from build123d import *

# Parameters (mm, degrees)
SKETCH1_W           = 422.275
SKETCH1_H           = 241.3
BOSS_EXTRUDE1_DEPTH = 19.05
CUT_EXTRUDE1_REACH  = 245.923
SKETCH2_W           = 231.775
SKETCH2_H           = 65.151
CUT_EXTRUDE2_REACH  = 323.197
SKETCH3_W           = 14.2875
SKETCH3_H           = 3.175
CUT_EXTRUDE3_REACH  = 323.197
SKETCH4_W           = 13.49375
SKETCH4_H           = 3.175
FILLET1_R           = 63.5
CUT_EXTRUDE4_REACH  = 323.197
SKETCH5_W           = 13.49375
SKETCH5_H           = 9.525
CHAMFER1_SIZE       = 3.175
CHAMFER1_SIZE2      = 11.849261314


with BuildPart() as part:
    # Sketch1 → Boss-Extrude1 (new body)
    with BuildSketch(Plane(origin=(0, 0, 0), x_dir=(1, 0, 0), z_dir=(0, 1, 0))):
        Rectangle(SKETCH1_W, SKETCH1_H)
    extrude(amount=BOSS_EXTRUDE1_DEPTH)

    # Sketch2 → Cut-Extrude1 (cut, up to next)
    with BuildSketch(Plane(origin=(0, 19.05, 0), x_dir=(1, 0, 0), z_dir=(0, 1, 0)), mode=Mode.PRIVATE) as cut_extrude1_sk1:
        with Locations((0, -88.0745)):
            Rectangle(SKETCH2_W, SKETCH2_H)
    cut_extrude1_tool1 = extrude(cut_extrude1_sk1.sketch, amount=-CUT_EXTRUDE1_REACH, mode=Mode.PRIVATE) & part.part
    add(cut_extrude1_tool1.solids().sort_by_distance((0, 19.05, 88.0745))[0], mode=Mode.SUBTRACT)

    # Sketch3 → Cut-Extrude2 (cut, up to next)
    with BuildSketch(Plane.XY.offset(120.65), mode=Mode.PRIVATE) as cut_extrude2_sk1:
        with Locations((-123.03125, 1.5875)):
            Rectangle(SKETCH3_W, SKETCH3_H)
    cut_extrude2_tool1 = extrude(cut_extrude2_sk1.sketch, amount=-CUT_EXTRUDE2_REACH, mode=Mode.PRIVATE) & part.part
    # Sketch3 → Cut-Extrude2 (cut, up to next)
    with BuildSketch(Plane.XY.offset(120.65), mode=Mode.PRIVATE) as cut_extrude2_sk2:
        with Locations((123.03125, 1.5875)):
            Rectangle(SKETCH3_W, SKETCH3_H)
    cut_extrude2_tool2 = extrude(cut_extrude2_sk2.sketch, amount=-CUT_EXTRUDE2_REACH, mode=Mode.PRIVATE) & part.part
    add(cut_extrude2_tool1.solids().sort_by_distance((-123.03125, 1.5875, 120.65))[0], mode=Mode.SUBTRACT)
    add(cut_extrude2_tool2.solids().sort_by_distance((123.03125, 1.5875, 120.65))[0], mode=Mode.SUBTRACT)

    # Sketch4 → Cut-Extrude3 (cut, up to next)
    with BuildSketch(Plane.XY.offset(120.65), mode=Mode.PRIVATE) as cut_extrude3_sk1:
        with Locations((-204.390625, 1.5875)):
            Rectangle(SKETCH4_W, SKETCH4_H)
    cut_extrude3_tool1 = extrude(cut_extrude3_sk1.sketch, amount=-CUT_EXTRUDE3_REACH, mode=Mode.PRIVATE) & part.part
    # Sketch4 → Cut-Extrude3 (cut, up to next)
    with BuildSketch(Plane.XY.offset(120.65), mode=Mode.PRIVATE) as cut_extrude3_sk2:
        with Locations((204.390625, 1.5875)):
            Rectangle(SKETCH4_W, SKETCH4_H)
    cut_extrude3_tool2 = extrude(cut_extrude3_sk2.sketch, amount=-CUT_EXTRUDE3_REACH, mode=Mode.PRIVATE) & part.part
    add(cut_extrude3_tool1.solids().sort_by_distance((-204.390625, 1.5875, 120.65))[0], mode=Mode.SUBTRACT)
    add(cut_extrude3_tool2.solids().sort_by_distance((204.390625, 1.5875, 120.65))[0], mode=Mode.SUBTRACT)

    # Fillet1
    fillet1_edges = [part.edges().sort_by_distance(p)[0] for p in [
        (211.1375, 11.1125, 120.65),
        (-211.1375, 11.1125, 120.65),
    ]]
    fillet(fillet1_edges, radius=FILLET1_R)

    # Sketch5 → Cut-Extrude4 (cut, up to next)
    with BuildSketch(Plane(origin=(0, 0, -120.65), x_dir=(-1, 0, 0), z_dir=(0, 0, -1)), mode=Mode.PRIVATE) as cut_extrude4_sk1:
        with Locations((-204.390625, 7.9375)):
            Rectangle(SKETCH5_W, SKETCH5_H)
    cut_extrude4_tool1 = extrude(cut_extrude4_sk1.sketch, amount=-CUT_EXTRUDE4_REACH, mode=Mode.PRIVATE) & part.part
    # Sketch5 → Cut-Extrude4 (cut, up to next)
    with BuildSketch(Plane(origin=(0, 0, -120.65), x_dir=(-1, 0, 0), z_dir=(0, 0, -1)), mode=Mode.PRIVATE) as cut_extrude4_sk2:
        with Locations((204.390625, 7.9375)):
            Rectangle(SKETCH5_W, SKETCH5_H)
    cut_extrude4_tool2 = extrude(cut_extrude4_sk2.sketch, amount=-CUT_EXTRUDE4_REACH, mode=Mode.PRIVATE) & part.part
    add(cut_extrude4_tool1.solids().sort_by_distance((204.390625, 7.9375, -120.65))[0], mode=Mode.SUBTRACT)
    add(cut_extrude4_tool2.solids().sort_by_distance((-204.390625, 7.9375, -120.65))[0], mode=Mode.SUBTRACT)

    # Chamfer1
    chamfer1_edges = [part.edges().sort_by_distance(p)[0] for p in [
        (0, 0, 55.499),
    ]]
    chamfer1_side = [part.faces().sort_by_distance(p)[0] for p in [
        (0, 9.525, 55.499),
    ]]
    chamfer(chamfer1_edges, length=CHAMFER1_SIZE, length2=CHAMFER1_SIZE2, reference=chamfer1_side[0])


solid = part.part
The model under review builds one solid part; all positions refer to its coordinate system, in mm. A direction names the side the tool comes from. Coordinates: 2 decimals unless noted, no trailing zeros. Order: outer loops, then holes, each group sorted by start corner. A loop starts at its lowest first (then second) coordinate and runs counter-clockwise, first axis right, second up. Notation, with made-up numbers: (71, -16) -> (124, -16) arc R35 cw to (124, 18) -> close; hole circle Ø7 at (-35.75, 80.25). An arc over 180 degrees is marked (long way). Answer in a Markdown table with one row per item.
(1) Consider section C-C (x = 14.5). Write out the cut boundary in (y, z) (3 decimals), plus the area to 3 significant figures.
Answers:
| item | result |
|---|---|
| outline | (0, -120.65) -> (19.05, -120.65) -> (19.05, 55.499) -> (3.175, 55.499) -> (0, 43.65) -> close |
| area | 3,340 mm² |
(2) Machinability: for faces 4 (the flat face through (115.888, 11, 89)), 5 (the flat face through (1.622, 1.565, 49.491)), 6 (the flat face through (123, 3.175, 2)), which of the approach directions +Z, -Z, +X, -X, +Y, -Y give a long, thin tool a straight path to every point of the face, cutting with its end or side? Answer none if there is none.
Answers:
| item | result |
|---|---|
| face 4 | +Z, +Y, -Y |
| face 5 | +Z, -Y |
| face 6 | +Z, -Z, -Y |
(3) Wall thickness on line 1 along X through (y, z) = (3, -30.5) (1 decimal); line 2 along Z through (x, y) = (-27, 9.25); line 3 along X through (y, z) = (6.25, -92): over which ranges is each line inside the solid? List them lowest first.
Answers:
| item | result |
|---|---|
| line 1 | -197.6 to -130.2, -115.9 to 115.9, 130.2 to 197.6 |
| line 2 | -120.65 to 55.5 |
| line 3 | -197.64 to 197.64 |
(4) Insertion check: pin 1 (6.5 mm diameter, centred on y = 4.5, z = -17, fed in from +X); pin 2 (1 mm diameter, centred on y = 16.5, z = 79, fed in from +X); pin 3 (4.5 mm diameter, centred on x = -123.5, z = -45, fed in from -Y) (3 decimals). Each pin has a flat end and moves straight along its axis. Give the tip position at first contact, or say it passes through.
Answers:
| item | result |
|---|---|
| pin 1 | x = 197.64 |
| pin 2 | x = 207.44 |
| pin 3 | y = 3.175 |
(5) Consider section B-B (y = 7.75). Write out the cut boundary in (x, z).
Answers:
| item | result |
|---|---|
| outline | (-197.64, -120.65) -> (197.64, -120.65) -> (197.64, 96.29) arc R63.5 ccw to (147.64, 120.65) -> (115.89, 120.65) -> (115.89, 55.5) -> (-115.89, 55.5) -> (-115.89, 120.65) -> (-147.64, 120.65) arc R63.5 ccw to (-197.64, 96.29) -> close |
(6) The part is to be moulded in two halves that separate along X. For faces 1 (the flat face through (-197.644, 6, -14)), 2 (the flat face through (-123, 3.175, 2)), 3 (the flat face through (163, 0, -2)), say which applies: +X half, -X half, draft (parallel to the pull), parting line (faces both ways), or undercut.
Answers:
| item | result |
|---|---|
| face 1 | -X half |
| face 2 | undercut |
| face 3 | draft |
